Could you check a few things on this model? Use its own coordinates, in mm. Face numbers are marked on the shaded views. Round coordinates to 2 decimals unless told otherwise and drop trailing zeros. Loops run counter-clockwise (first coordinate to the right, second up) from the corner with the lowest first, then second, coordinate; pieces in that order, holes last. Notation, with made-up numbers: M -8,-0.75 L -2,-0.75 A16 cw -2,17.25 Z; hole C -19.5,23 d1. An arc over 180 degrees is marked long. Answer in a Markdown table with one row per item.
```python
from build123d import *

# Parameters (mm, degrees)
SKETCH1_R           = 35
SKETCH1_R_2         = 6.1
SKETCH1_R_3         = 4
BOSS_EXTRUDE2_DEPTH = 5
FILLET1_R           = 0.25


with BuildPart() as part:
    # Sketch1 → Boss-Extrude2 (new body)
    with BuildSketch(Plane(origin=(0, 0, 0), x_dir=(1, 0, 0), z_dir=(0, 1, 0))):
        Circle(SKETCH1_R)
        Circle(SKETCH1_R_2, mode=Mode.SUBTRACT)
        with Locations((-23.61, 0)):
            Circle(SKETCH1_R_3, mode=Mode.SUBTRACT)
        with Locations((0, -25.5)):
            Circle(SKETCH1_R_3, mode=Mode.SUBTRACT)
    extrude(amount=BOSS_EXTRUDE2_DEPTH)

    # Fillet1
    fillet1_edges = [part.edges().sort_by_distance(p)[0] for p in [
        (-35, 5, 0),
    ]]
    fillet(fillet1_edges, radius=FILLET1_R)


solid = part.part
```
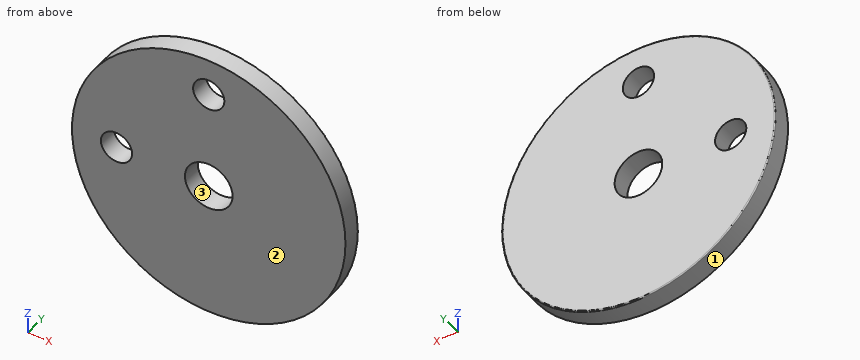
1) I want a section at A-A, the plane x = 0. Please give me the cut outline in (y, z), plus the area to 3 significant figures.
Computed:
| item | result |
|---|---|
| outline | M 0,-35 L 4.75,-35 A0.25 ccw 5,-34.75 L 5,-6.1 L 0,-6.1 Z; M 0,6.1 L 5,6.1 L 5,21.5 L 0,21.5 Z; M 0,29.5 L 5,29.5 L 5,34.75 A0.25 ccw 4.75,35 L 0,35 Z |
| area | 249 mm² |
2) If we mould it in two halves opening along X, with no side actions, what happens to the marked faces 1, 2 and 3? For each: released by +X, released by -X, zero draft, split by the parting line, or undercut.
Computed:
| item | result |
|---|---|
| face 1 | split by the parting line |
| face 2 | zero draft |
| face 3 | undercut |
3) I want a section at C-C, the plane y = 3. Please give me the cut outline in (x, z).
Computed:
| item | result |
|---|---|
| outline | C 0,0 d70; hole C -23.61,0 d8; hole C 0,0 d12.2; hole C 0,25.5 d8 |
4) I want a section at B-B, the plane z = 0. Please give me the cut outline in (x, y), plus the area to 3 significant figures.
Computed:
| item | result |
|---|---|
| outline | M -35,0 L -27.61,0 L -27.61,5 L -34.75,5 A0.25 ccw -35,4.75 Z; M -19.61,0 L -6.1,0 L -6.1,5 L -19.61,5 Z; M 6.1,0 L 35,0 L 35,4.75 A0.25 ccw 34.75,5 L 6.1,5 Z |
| area | 249 mm² |
5) Will these pins go through, and if not, where does the flat tip stop? P1, Ø1, axis at y = 3, z = -7, coming from the -X side; P2, Ø1, axis at x = -17.5, y = 2, coming from the +Z side; P3, Ø1, axis at x = 9, y = 2, coming from the -Z side.
Computed:
| item | result |
|---|---|
| P1 | stops at x = -34.39 |
| P2 | stops at z = 30.59 |
| P3 | stops at z = -33.95 |
6) I need wall thicknesses on line 1 (Z direction, x = 0, y = 1.4); line 2 (X direction, y = 1.5, z = 0); line 3 (X direction, y = 2.3, z = 2). Which ranges of each line are inside material? Lowest first, please.
Computed:
| item | result |
|---|---|
| line 1 | z = -35 to -6.1, 6.1 to 21.5, 29.5 to 35 |
| line 2 | x = -35 to -27.61, -19.61 to -6.1, 6.1 to 35 |
| line 3 | x = -34.94 to -27.07, -20.15 to -5.76, 5.76 to 34.94 |
